The drawing under review shows one solid part. Ordinate dimensions are in mm from its lowest x, y, z. Coordinates: 2 decimals unless noted, no trailing zeros. Write each loop counter-clockwise with the first axis right and the second up, starting at its lowest first coordinate (ties: lowest second). Pieces come first, ordered by that corner, then holes.
Q1. Take a section at D-D (z = 0.5). Give the boundary of the cut face in (x, y) (3 decimals).
Q2. Take a section at B-B (z = 2.5). Give the boundary of the cut face in (x, y) (3 decimals).
Q3. Take a section at C-C (y = 3.7). Give the boundary of the cut face in (x, z), and give its area (3 significant figures).
Q4. Mouldability with a two-part tool opening along X and no side actions: class the marked faces 1, 2 and 3 as pulls with the +X half, pulls with the -X half, needs draft (parallel to the pull), parting line crosses it, or undercut.
Q5. Take a section at A-A (x = 2.4). Give the boundary of the cut face in (y, z), and give its area (3 significant figures).
Q6. Insertion check: pin 1 (3 mm diameter, centred on x = 7.5, z = 4.5, fed in from -Y). The pin has a flat end and moves straight along its axis. Give the tip position at first contact, or say it passes through.
Q7. For probe 1 along X at (y, z) = (3, 1.6); probe 2 along X at (y, z) = (0.6, 2.5); probe 3 along Z at (x, y) = (2.4, 3.4), list the stretches that pass through material, from the lowest coordinate up.
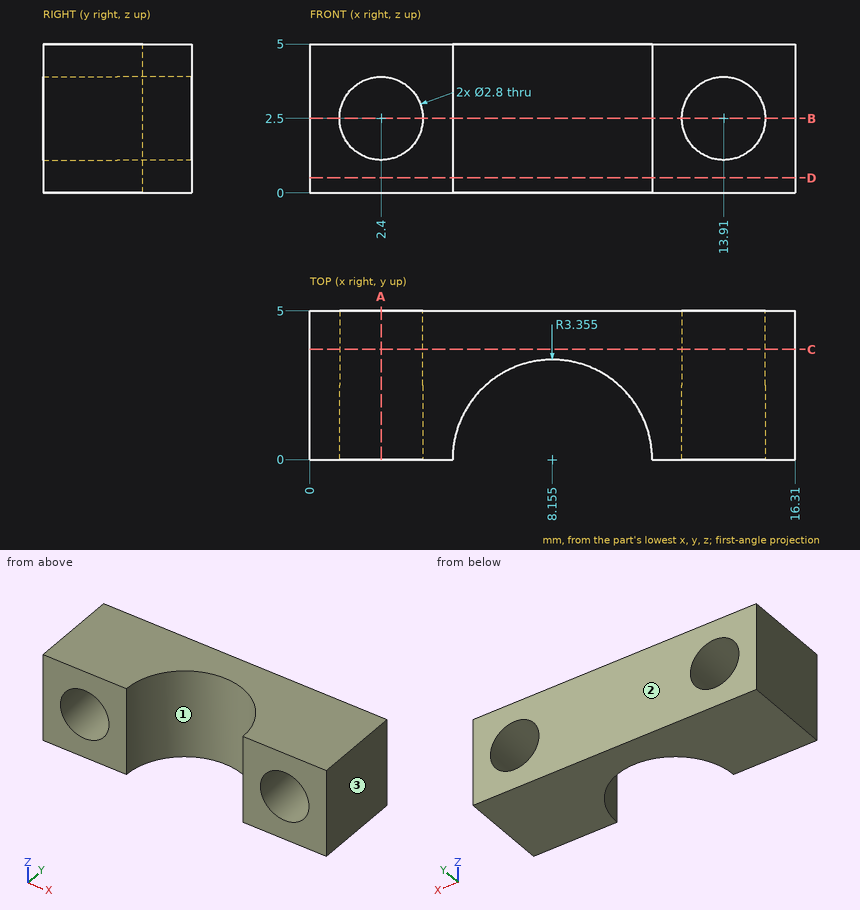
Response:
1. outline: (0, 0) - (4.8, 0) arc R3.355 cw to (11.51, 0) - (16.31, 0) - (16.31, 5) - (0, 5) - close
2. outline: (0, 0) - (1, 0) - (1, 5) - (0, 5) - close; (3.8, 0) - (4.8, 0) arc R3.355 cw to (11.51, 0) - (12.51, 0) - (12.51, 5) - (3.8, 5) - close; (15.31, 0) - (16.31, 0) - (16.31, 5) - (15.31, 5) - close
3. outline: (0, 0) - (16.31, 0) - (16.31, 5) - (0, 5) - close; hole circle Ø2.8 at (2.4, 2.5); hole circle Ø2.8 at (13.91, 2.5)
3. area: 69.2 mm2
4. face 1: undercut
4. face 2: needs draft
4. face 3: pulls with the +X half
5. outline: (0, 0) - (5, 0) - (5, 1.1) - (0, 1.1) - close; (0, 3.9) - (5, 3.9) - (5, 5) - (0, 5) - close
5. area: 11.0 mm2
6. pin 1: stops at y = 2.57
7. probe 1: x = 0 to 1.33, 3.47 to 6.65, 9.66 to 12.84, 14.98 to 16.31
7. probe 2: x = 0 to 1, 3.8 to 4.85, 11.46 to 12.51, 15.31 to 16.31
7. probe 3: z = 0 to 1.1, 3.9 to 5
